Here's how the part is built. I have some questions about the finished solid (model axes, mm). Face numbers are marked on the shaded views. Coordinates: 2 decimals unless noted, no trailing zeros. Loops run counter-clockwise (first coordinate to the right, second up) from the corner with the lowest first, then second, coordinate; pieces in that order, holes last. Notation, with made-up numbers: (36, -31.75) -> (95, -31.75) arc R17 cw to (95, -21.75) -> close; hole circle Ø5 at (34, 43). An arc over 180 degrees is marked (long way). Answer as a JSON object with one key per item and string values. Group by question number.
1) If we mould it in two halves opening along Z, with no side actions, what happens to the marked faces 1, 2 and 3? For each: +Z half, -Z half, draft (parallel to the pull), parting line (faces both ways), or undercut.
2) I'm going to push flat-ended pins straight in: pin 1 (5.5 mm diameter, centred on y = 5, z = 356, fed in from +X); pin 2 (4 mm diameter, centred on x = 26.5, y = 2.5, fed in from -Z); pin 3 (1.5 mm diameter, centred on x = 5, z = 320, fed in from +Y); pin 4 (23 mm diameter, centred on x = 6, y = -7, fed in from -Z). Where does each tip first touch, or does it pass through?
3) I want a section at B-B (x = -24.5). Write out the boundary of the cut face in (y, z).
4) I want a section at D-D (z = 216). Write out the boundary of the cut face in (x, y).
5) I want a section at A-A (z = 314). Write out the boundary of the cut face in (x, y), then the cut area to 3 significant figures.
6) I need wall thicknesses on probe 1 along Z at (x, y) = (12.5, -20); probe 2 along X at (y, z) = (-34.5, 69); probe 3 along Y at (x, z) = (13, 33.5). Which ranges of each line are inside material? Lowest first, please. Write a range as [from, to].
7) I want a section at C-C (y = 33.5). Write out the boundary of the cut face in (x, z), then the cut area to 3 significant figures.
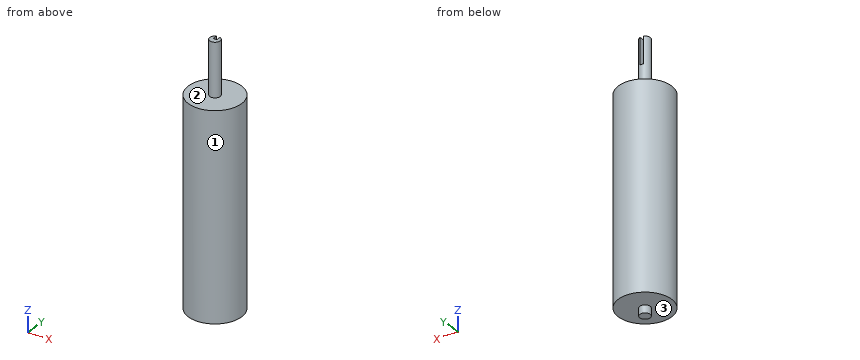
```python
from build123d import *

# Parameters (mm, degrees)
SKETCH1_R               = 38.1
BOSS_EXTRUDE1_DEPTH     = 292.1
SKETCH3_R               = 7.5
BOSS_EXTRUDE2_DEPTH     = 76.2
CUT_EXTRUDE1_DEPTH      = 1
CUT_EXTRUDE1_DEPTH_BACK = 38.1
SKETCH5_R               = 7.5
BOSS_EXTRUDE3_DEPTH     = 11


with BuildPart() as part:
    # Sketch1 → Boss-Extrude1 (new body)
    with BuildSketch(Plane.XY):
        Circle(SKETCH1_R)
    extrude(amount=BOSS_EXTRUDE1_DEPTH)

    # Sketch3 → Boss-Extrude2 (add)
    with BuildSketch(Plane.XY.offset(292.1)):
        Circle(SKETCH3_R)
    extrude(amount=BOSS_EXTRUDE2_DEPTH)

    # Sketch4 → Cut-Extrude1 (cut, two sides)
    with BuildSketch(Plane.XY.offset(368.3)) as cut_extrude1_sk:
        Polygon((-2.5, 138.541811076), (-2.5, 7.071067812), (-2.5, 0), (2.5, 0), (2.5, 7.071067812), (2.5, 138.541811076), (2.5, 401.483297603), (-2.5, 401.483297603), align=None)
    extrude(amount=CUT_EXTRUDE1_DEPTH, mode=Mode.SUBTRACT)
    extrude(cut_extrude1_sk.sketch, amount=-CUT_EXTRUDE1_DEPTH_BACK, mode=Mode.SUBTRACT)

    # Sketch5 → Boss-Extrude3 (add)
    with BuildSketch(Plane(origin=(0, 0, 0), x_dir=(-1, 0, 0), z_dir=(0, 0, -1))):
        Circle(SKETCH5_R)
    extrude(amount=BOSS_EXTRUDE3_DEPTH)


solid = part.part
```
Determined:
{
 "1": {"face 1": "draft", "face 2": "+Z half", "face 3": "-Z half"},
 "2": {"pin 1": "x = 7.15", "pin 2": "z = 0", "pin 3": "y = 6.18", "pin 4": "z = -11"},
 "3": {"outline": "(-29.18, 0) -> (29.18, 0) -> (29.18, 292.1) -> (-29.18, 292.1) -> close"},
 "4": {"outline": "circle Ø76.2 at (0, 0)"},
 "5": {"outline": "circle Ø15 at (0, 0)", "area": "177 mm^2"},
 "6": {"probe 1": "[0, 292.1]", "probe 2": "[-16.17, 16.17]", "probe 3": "[-35.81, 35.81]"},
 "7": {"outline": "(-18.15, 0) -> (18.15, 0) -> (18.15, 292.1) -> (-18.15, 292.1) -> close", "area": "10,600 mm^2"}
}
